Here's how the part is built. I have some questions about the finished solid (model axes, mm). A direction names the side the tool comes from. Coordinates: 2 decimals unless noted, no trailing zeros. Write each loop counter-clockwise with the first axis right and the second up, starting at its lowest first coordinate (ties: lowest second). Pieces come first, ordered by that corner, then holes. Notation, with made-up numbers: (-28.5, 34) -> (22.5, 34) arc R27 cw to (22.5, 59) -> close; hole circle Ø9 at (42, 74.25). An arc over 180 degrees is marked (long way). Use a Markdown table: item, result. Add a question column.
Autodesk Inventor part; units mm, degrees
ref_plane "YZ Plane" through (0, 0, 0) normal (1, 0, 0) x (0, 1, 0)
ref_plane "XZ Plane" through (0, 0, 0) normal (0, 1, 0) x (-1, 0, 0)
ref_plane "XY Plane" through (0, 0, 0) normal (0, 0, 1) x (1, 0, 0)
sketch "Sketch1" plane through (0, 0, 0) normal (0, 0, 1) x (1, 0, 0)
  circle A0 centre (-414.4261, -56.251) radius 4.7625
  point P0 (0, 0)
  dimension "d0" = 9.525
extrude "Extrusion1" add sketch "Sketch1" against normal blind 25.4
sketch "Sketch2" plane through (-414.4261, -56.251, 0) normal (0, 0, 1) x (1, 0, 0)
  circle A0 centre (0, 0) radius 4.7625
  line L0 (-8.2489, 0) -> (-4.1244, 7.1437)
  line L1 (-4.1244, 7.1437) -> (4.1244, 7.1438)
  line L2 (4.1244, 7.1438) -> (8.2489, 0)
  line L3 (8.2489, 0) -> (4.1244, -7.1437)
  line L4 (4.1244, -7.1437) -> (-4.1244, -7.1438)
  line L5 (-4.1244, -7.1438) -> (-8.2489, 0)
  point P0 (414.4261, 56.251)
  dimension "d3" = 14.2875
extrude "Extrusion2" add sketch "Sketch2" along normal blind 3.175 contours A0 | L0 L1 L2 L3 L4 L5
thread "Thread1"
chamfer "Chamfer1" distance 0.508 angle 45 1 edges at (-419.1886, -56.251, -25.4)
properties part number "375 bolt x4" material "Steel"
Q1. Thinking about a two-plate mould opening in Y: for faces 3 (the flat face through (-408.27, -52.63, 1.57)), 4 (the cylindrical face through (-419.184, -56.042, -12.272)), 5 (the flat face through (-414, -56, -25.4)), 6 (the flat face through (-408.21, -59.77, 1.57)), which applies, released by +Y, released by -Y, zero draft, split by the parting line, or undercut?
Q2. Will these pins go through, and if not, where does the flat tip stop? pin 1 (4 mm diameter, centred on y = -57.5, z = -15.5, fed in from -X); pin 2 (3 mm diameter, centred on y = -51, z = -9.5, fed in from +X).
Q3. Suppose I cut it at C-C, the plane z = -14.5. Write out the boundary of the cut face in (x, y) (1 decimal).
Q4. Suppose I cut it at A-A, the plane z = 1. Write out the boundary of the cut face in (x, y) (1 decimal), and give its area (3 significant figures).
Q5. Suppose I cut it at B-B, the plane x = -421. Write out the boundary of the cut face in (y, z) (3 decimals).
Q6. Please list where these lines run through material, in increasing order: line 1 (Z direction, x = -410.5, y = -53.5) (3 decimals); line 2 (X direction, y = -56, z = -20.25); line 3 (X direction, y = -58.25, z = -12).
Q7. Which directions (+Z, -Z, +X, -X, +Y, -Y) give clear straight access to the entire face, cutting with the end or side of a thin tool? Please do faces 1 (the flat face through (-420.584, -59.873, 1.565)), 2 (the flat face through (-415, -51, 0)).
Answer key:
| question | item | result |
|---|---|---|
| 1 | face 3 | released by +Y |
| 1 | face 4 | split by the parting line |
| 1 | face 5 | zero draft |
| 1 | face 6 | released by -Y |
| 2 | pin 1 | stops at x = -419.19 |
| 2 | pin 2 | stops at x = -411.49 |
| 3 | outline | circle Ø9.5 at (-414.4, -56.3) |
| 4 | outline | (-422.7, -56.3) -> (-418.6, -63.4) -> (-410.3, -63.4) -> (-406.2, -56.3) -> (-410.3, -49.1) -> (-418.6, -49.1) -> close |
| 4 | area | 177 mm^2 |
| 5 | outline | (-59.152, 0) -> (-53.35, 0) -> (-53.35, 3.175) -> (-59.152, 3.175) -> close |
| 6 | line 1 | z = 0 to 3.175 |
| 6 | line 2 | x = -419.18 to -409.67 |
| 6 | line 3 | x = -418.75 to -410.1 |
| 7 | face 1 | +Z, -Z, -X, -Y |
| 7 | face 2 | -Z |
